Here's the drawing with two shaded views (mm, measured from the low corner). I have some questions. Give positions to 0.01 mm unless a question says otherwise; leave off trailing zeros. Write each loop counter-clockwise with the first axis right and the second up, starting at its lowest first coordinate (ties: lowest second). Pieces come first, ordered by that corner, then holes. Notation, with made-up numbers: (38, -20) -> (87, -20) arc R16 ccw to (87, -11) -> close; hole circle Ø6 at (81, 64). An arc over 180 degrees is marked (long way). One line per item, written item: value.
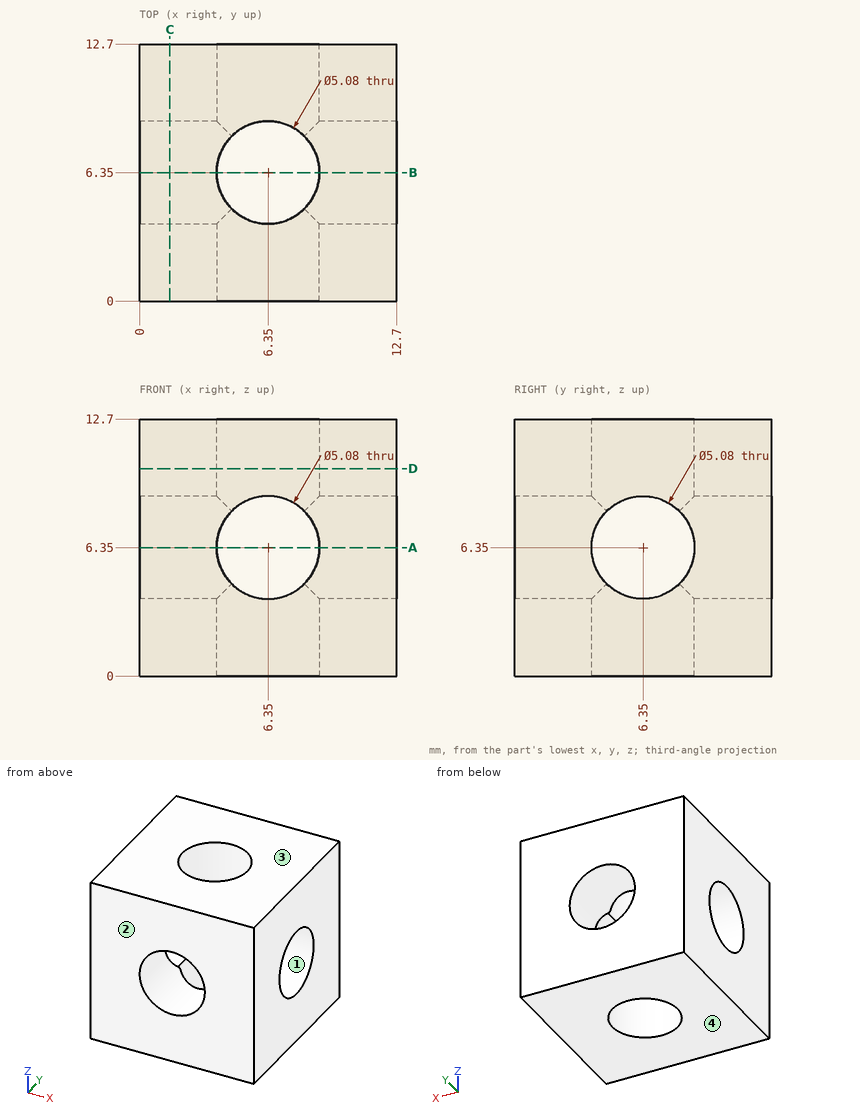
1) We'd pull the mould along Z, two halves only. Please class the marked faces 1, 2, 3 and 4: released by +Z, released by -Z, zero draft, split by the parting line, or undercut.
Answer list:
face 1: undercut
face 2: zero draft
face 3: released by +Z
face 4: released by -Z
2) If we section it at C-C (x = 1.5): Write out the boundary of the cut face in (y, z).
Answer list:
outline: (0, 0) -> (12.7, 0) -> (12.7, 12.7) -> (0, 12.7) -> close; hole circle Ø5.08 at (6.35, 6.35)
3) I need wall thicknesses on L1, parallel to Z at x = 9.1, y = 6.35. Which ranges of the line are inside material? Lowest first, please.
Answer list:
L1: z = 0 to 3.81, 8.89 to 12.7
4) If we section it at A-A (z = 6.35): Write out the boundary of the cut face in (x, y).
Answer list:
outline: (0, 0) -> (3.81, 0) -> (3.81, 3.81) -> (0, 3.81) -> close; (0, 8.89) -> (3.81, 8.89) -> (3.81, 12.7) -> (0, 12.7) -> close; (8.89, 0) -> (12.7, 0) -> (12.7, 3.81) -> (8.89, 3.81) -> close; (8.89, 8.89) -> (12.7, 8.89) -> (12.7, 12.7) -> (8.89, 12.7) -> close
